Check sheet for the modelled part. Datum: model origin and axes. Units: mm. A direction names the side the tool comes from. Give positions to 0.01 mm unless a question says otherwise; leave off trailing zeros. Loops run counter-clockwise (first coordinate to the right, second up) from the corner with the lowest first, then second, coordinate; pieces in that order, holes last. Notation, with made-up numbers: M 57.5,34 L 90.5,34 A22 ccw 90.5,53 Z; hole C 42,18 d4. An arc over 180 degrees is marked long. Use one line per item in the form item = value.
from build123d import *

# Parameters (mm, degrees)
BOSS_EXTRUDE1_DEPTH = 7.5
SKETCH2_R           = 10
CUT_EXTRUDE1_DEPTH  = 8.5
SKETCH3_W           = 16.45751311
SKETCH3_H           = 74.99964242
CUT_EXTRUDE2_DEPTH  = 5
FILLET2_R           = 2
FILLET3_R           = 2
FILLET4_R           = 2
BOSS_EXTRUDE2_DEPTH = 15
SKETCH8_R           = 5
CUT_EXTRUDE3_DEPTH  = 171


with BuildPart() as part:
    # Sketch1 → Boss-Extrude1 (new body)
    with BuildSketch(Plane.XY):
        with BuildLine():
            Line((-13.228756555, -15), (-13.228756555, -85.952171431))
            ThreePointArc((-13.228756555, -85.952171431), (-17.096585846, -105.234879374), (-28.10166958, -121.534298414))
            ThreePointArc((-28.10166958, -121.534298414), (-36.905736568, -134.573833645), (-40, -150))
            Line((-40, -150), (-25, -150))
            ThreePointArc((-25, -150), (-17.67766953, -132.32233047), (0, -125))
            ThreePointArc((0, -125), (17.67766953, -132.32233047), (25, -150))
            Line((25, -150), (40, -150))
            ThreePointArc((40, -150), (36.905736568, -134.573833645), (28.10166958, -121.534298414))
            ThreePointArc((28.10166958, -121.534298414), (17.096585846, -105.234879374), (13.228756555, -85.952171431))
            Line((13.228756555, -85.952171431), (13.228756555, -15))
            ThreePointArc((13.228756555, -15), (0, 20), (-13.228756555, -15))
        make_face()
    extrude(amount=BOSS_EXTRUDE1_DEPTH)

    # Sketch2 → Cut-Extrude1 (cut, through all)
    with BuildSketch(Plane.XY.offset(7.5)):
        Circle(SKETCH2_R)
    extrude(amount=-CUT_EXTRUDE1_DEPTH, mode=Mode.SUBTRACT)

    # Sketch3 → Cut-Extrude2 (cut)
    with BuildSketch(Plane.XY.offset(7.5)):
        with Locations((0, -67.5)):
            Rectangle(SKETCH3_W, SKETCH3_H)
    extrude(amount=-CUT_EXTRUDE2_DEPTH, mode=Mode.SUBTRACT)

    # Fillet2
    fillet2_edges = [part.edges().sort_by_distance(p)[0] for p in [
        (8.228756555, -30.00017879, 5),
        (0, -104.99982121, 2.5),
        (8.228756555, -104.99982121, 5),
        (-8.228756555, -104.99982121, 5),
        (0, -30.00017879, 2.5),
        (-8.228756555, -30.00017879, 5),
        (8.228756555, -67.5, 7.5),
        (0, -30.00017879, 7.5),
        (-8.228756555, -67.5, 7.5),
        (0, -104.99982121, 7.5),
    ]]
    fillet(fillet2_edges, radius=FILLET2_R)

    # Mirror1: part across plane


with BuildPart() as part_1:
    add(part.part)
    add(part.part.mirror(Plane(origin=(-63.228756555, -85.952171431, 0), x_dir=(1, 0, 0), z_dir=(0, 0, 1))))

    # Fillet3
    fillet3_edges = [part_1.edges().sort_by_distance(p)[0] for p in [
        (-10, 0, 7.5),
    ]]
    fillet(fillet3_edges, radius=FILLET3_R)

    # Fillet4
    fillet4_edges = [part_1.edges().sort_by_distance(p)[0] for p in [
        (-10, 0, -7.5),
    ]]
    fillet(fillet4_edges, radius=FILLET4_R)

    # Sketch7 → Boss-Extrude2 (add)
    with BuildSketch(Plane.XY.offset(7.5)):
        with BuildLine():
            Line((-40, -150), (-40, -125))
            ThreePointArc((-40, -125), (-26.219237737, -117.816300802), (-17.096585846, -105.234879374))
            ThreePointArc((-17.096585846, -105.234879374), (-21.789831556, -113.931011558), (-28.10166958, -121.534298414))
            ThreePointArc((-28.10166958, -121.534298414), (-36.905736568, -134.573833645), (-40, -150))
        make_face()
        with BuildLine():
            Line((40, -150), (40, -125))
            ThreePointArc((40, -125), (26.219237737, -117.816300802), (17.096585846, -105.234879374))
            ThreePointArc((17.096585846, -105.234879374), (21.789831556, -113.931011558), (28.10166958, -121.534298414))
            ThreePointArc((28.10166958, -121.534298414), (36.905736568, -134.573833645), (40, -150))
        make_face()
    extrude(amount=-BOSS_EXTRUDE2_DEPTH)

    # Sketch8 → Cut-Extrude3 (cut, through all)
    with BuildSketch(Plane(origin=(0, -150, 0), x_dir=(-1, 0, 0), z_dir=(0, -1, 0))):
        with Locations((32.5, 0)):
            Circle(SKETCH8_R)
        with Locations((-32.5, 0)):
            Circle(SKETCH8_R)
    extrude(amount=-CUT_EXTRUDE3_DEPTH, mode=Mode.SUBTRACT)


solid = part_1.part
1) Section check D-D (x = -32.5). Record the cut outline in (y, z).
Evaluation:
outline = M -150,-7.5 L -122.11,-7.5 L -122.11,-5 L -150,-5 Z; M -150,5 L -122.11,5 L -122.11,7.5 L -150,7.5 Z
2) Scan lines: line 1 (X direction, y = -135, z = 0); line 2 (X direction, y = -129, z = 0); line 3 (Z direction, x = 32.5, y = -128.5). Record each from-to range of solid material in increasing order.
Evaluation:
line_1 = -40 to -37.5, -27.5 to -20, 20 to 27.5, 37.5 to 40
line_2 = -40 to -37.5, -27.5 to -13.56, 13.56 to 27.5, 37.5 to 40
line_3 = -7.5 to -5, 5 to 7.5
3) Depth check by flat-ended pin: pin 1 Ø9 at (x, z) = (-32.5, 0) entering from -Y; pin 2 Ø2 at (x, z) = (21.5, -2.5) entering from -Y; pin 3 Ø4.5 at (y, z) = (-60, 3.5) entering from +X; pin 4 Ø13 at (x, y) = (-2.5, -55.5) entering from +Z. Enter the tip coordinate at first touch or a pass-through.
Evaluation:
pin_1 = through
pin_2 = -139.1
pin_3 = 13.23
pin_4 = 7.08
4) Release check for a two-part mould opening along X. For faces 5 (the face through (-8.229, -68, 4)), 6 (the face through (13.229, -51, 0)), 7 (the face through (27, -150, 0)), 8 (the face through (-14.18, -95.65, 0.11)) record: pulls with the +X half, pulls with the -X half, needs draft (parallel to the pull), parting line crosses it, or undercut.
Evaluation:
face_5 = undercut
face_6 = pulls with the +X half
face_7 = needs draft
face_8 = pulls with the -X half
5) Section check A-A (x = 0). Record the cut outline in (y, z).
Evaluation:
outline = M -125,-7.5 L -107,-7.5 A2 ccw -105,-5.5 L -105,-4.5 A2 cw -103,-2.5 L -32,-2.5 A2 cw -30,-4.5 L -30,-5.5 A2 ccw -28,-7.5 L -12,-7.5 A2 ccw -10,-5.5 L -10,5.5 A2 ccw -12,7.5 L -28,7.5 A2 ccw -30,5.5 L -30,4.5 A2 cw -32,2.5 L -103,2.5 A2 cw -105,4.5 L -105,5.5 A2 ccw -107,7.5 L -125,7.5 Z; M 10,-5.5 A2 ccw 12,-7.5 L 20,-7.5 L 20,7.5 L 12,7.5 A2 ccw 10,5.5 Z
6) Section check C-C (y = -56). Record the cut outline in (x, z), then the cut area to 3 significant figures.
Evaluation:
outline = M -13.23,-7.5 L -10.23,-7.5 A2 ccw -8.23,-5.5 L -8.23,-2.5 L 8.23,-2.5 L 8.23,-5.5 A2 ccw 10.23,-7.5 L 13.23,-7.5 L 13.23,7.5 L 10.23,7.5 A2 ccw 8.23,5.5 L 8.23,2.5 L -8.23,2.5 L -8.23,5.5 A2 ccw -10.23,7.5 L -13.23,7.5 Z
area = 229 mm^2
7) Set-up check for faces 1 (the face through (23.854, -115.567, 0.105)), 2 (the face through (-8.229, -68, -4)), 3 (the face through (8.229, -68, 4)), 4 (the face through (-23.854, -115.567, 0.105)): record each of +Z, -Z, +X, -X, +Y, -Y from which the full face is reachable in a straight line by a thin tool's end or side.
Evaluation:
face_1 = +Z, -Z, +X
face_2 = -Z
face_3 = +Z
face_4 = +Z, -Z, -X
8) Section check B-B (y = 0). Record the cut outline in (x, z), then the cut area to 3 significant figures.
Evaluation:
outline = M -20,-7.5 L -12,-7.5 A2 ccw -10,-5.5 L -10,5.5 A2 ccw -12,7.5 L -20,7.5 Z; M 10,-5.5 A2 ccw 12,-7.5 L 20,-7.5 L 20,7.5 L 12,7.5 A2 ccw 10,5.5 Z
area = 297 mm^2
